Design review of the part built by this model. Coordinates are the model's own, in mm. A direction names the side the tool comes from. Round coordinates to 2 decimals unless told otherwise and drop trailing zeros. Loops run counter-clockwise (first coordinate to the right, second up) from the corner with the lowest first, then second, coordinate; pieces in that order, holes last. Notation, with made-up numbers: (5.25, 17) - (53.25, 17) arc R26 ccw to (53.25, 36) - close; hole circle Ø3 at (9, -6). An arc over 180 degrees is marked (long way). Return JSON: item names as keys, results as strings. Group by question number.
(1) The part is to be moulded in two halves that separate along Z. For faces 1 (the flat face through (23, 0, 0)), 2 (the flat face through (30, 0, 11)), 3 (the cylindrical face through (25.6, 0.02, 7.43)), say which applies: pulls with the +Z half, pulls with the -Z half, needs draft (parallel to the pull), parting line crosses it, or undercut.
(2) Clearance check with flat-ended pins moving along their axes: pin 1 (0.9 mm diameter, centred on x = -24, y = -0.5, fed in from -Z); pin 2 (1.5 mm diameter, centred on y = 0.5, z = -7, fed in from +X); pin 3 (1.5 mm diameter, centred on y = 0.5, z = 2, fed in from -X); pin 4 (1 mm diameter, centred on y = 0, z = 9.5, fed in from -X). State where each tip first meets the part, or that it passes through.
(3) We need section C-C, the plane z = -4.25. Write out the cut boundary in (x, y), and give its area (3 significant figures).
(4) We need section A-A, the plane x = 23.5. Write out the cut boundary in (y, z), and give its area (3 significant figures).
(5) For faces 4 (the flat face through (-23, 0, -0.853)), 5 (the flat face through (25, 0, -8)), 6 (the flat face through (-25, 0, 3)), list the 3-axis set-ups (+Z, -Z, +X, -X, +Y, -Y) from which the entire face can be reached by the end or side of a thin tool; tool diameter is ignored.
(6) Wall thickness on L1, parallel to X at y = 0.4, z = -1.5: over which ranges is the line inside the solid? List them lowest first. Write a range as [from, to].
from build123d import *

# Parameters (mm, degrees)
BOSS_EXTRUDE1_DEPTH     = 1.5
CUT_EXTRUDE1_DEPTH      = 34.674916481
CUT_EXTRUDE1_DEPTH_BACK = 34.674916481
FILLET1_R               = 2
FILLET2_R               = 0.5


with BuildPart() as part:
    # Sketch1 → Boss-Extrude1 (new, symmetric)
    with BuildSketch(Plane(origin=(0, 0, 0), x_dir=(1, 0, 0), z_dir=(0, 1, 0))):
        Polygon((-25, -15), (-30, -15), (-30, -8), (-25, -8), (-25, 15), (25, 15), (25, -8), (30, -8), (30, -15), (25, -15), align=None)
    extrude(amount=BOSS_EXTRUDE1_DEPTH, both=True)

    # Sketch2 → Cut-Extrude1 (cut, two sides: drawn at the far end of the back side and taken through both)
    with BuildSketch(Plane(origin=(0, 1.5, 0), x_dir=(1, 0, 0), z_dir=(0, 1, 0)).offset(-CUT_EXTRUDE1_DEPTH_BACK)):
        with BuildLine():
            Line((-25, 14.146806682), (-22, 14.146806682))
            Line((-22, 14.146806682), (-22, 15))
            Line((-22, 15), (-25, 15))
            ThreePointArc((-25, 15), (-30.216117819, 7.5), (-25, 0))
            Line((-25, 0), (-22, 0))
            Line((-22, 0), (-22, 0.853193318))
            Line((-22, 0.853193318), (-25, 0.853193318))
            ThreePointArc((-25, 0.853193318), (-29.422367819, 7.5), (-25, 14.146806682))
        make_face()
        with BuildLine():
            Line((22, 0.853193318), (22, 0))
            Line((22, 0), (25, 0))
            ThreePointArc((25, 0), (30.216117819, 7.5), (25, 15))
            Line((25, 15), (22, 15))
            Line((22, 15), (22, 14.146806682))
            Line((22, 14.146806682), (25, 14.146806682))
            ThreePointArc((25, 14.146806682), (29.422367819, 7.5), (25, 0.853193318))
            Line((25, 0.853193318), (22, 0.853193318))
        make_face()
    extrude(amount=CUT_EXTRUDE1_DEPTH + CUT_EXTRUDE1_DEPTH_BACK, mode=Mode.SUBTRACT)

    # Fillet1
    fillet1_edges = [part.edges().sort_by_distance(p)[0] for p in [
        (25, 0, 8),
        (30, 0, 8),
        (30, 0, 15),
        (-30, 0, 15),
        (-30, 0, 8),
        (-25, 0, 8),
    ]]
    fillet(fillet1_edges, radius=FILLET1_R)

    # Fillet2
    fillet2_edges = [part.edges().sort_by_distance(p)[0] for p in [
        (-25, 0, -14.146806682),
        (-25, 0, -0.853193318),
        (25, 0, -14.146806682),
        (25, 0, -0.853193318),
        (-22, 0, -15),
        (22, 0, -15),
    ]]
    fillet(fillet2_edges, radius=FILLET2_R)


solid = part.part
Solutions:
{
 "1": {"face 1": "undercut", "face 2": "needs draft", "face 3": "pulls with the -Z half"},
 "2": {"pin 1": "z = -14.15", "pin 2": "x = 25", "pin 3": "x = -25", "pin 4": "x = -30"},
 "3": {"outline": "(-25, -1.5) - (25, -1.5) - (25, 1.5) - (-25, 1.5) - close", "area": "150 mm^2"},
 "4": {"outline": "(-1.5, -14.15) - (1.5, -14.15) - (1.5, -0.85) - (-1.5, -0.85) - close; (-1.5, 0) - (1.5, 0) - (1.5, 15) - (-1.5, 15) - close", "area": "84.9 mm^2"},
 "5": {"face 4": "-X, +Y, -Y", "face 5": "-Z, +X, +Y, -Y", "face 6": "-Z, -X, +Y, -Y"},
 "6": {"L1": "[-25, 25]"}
}
